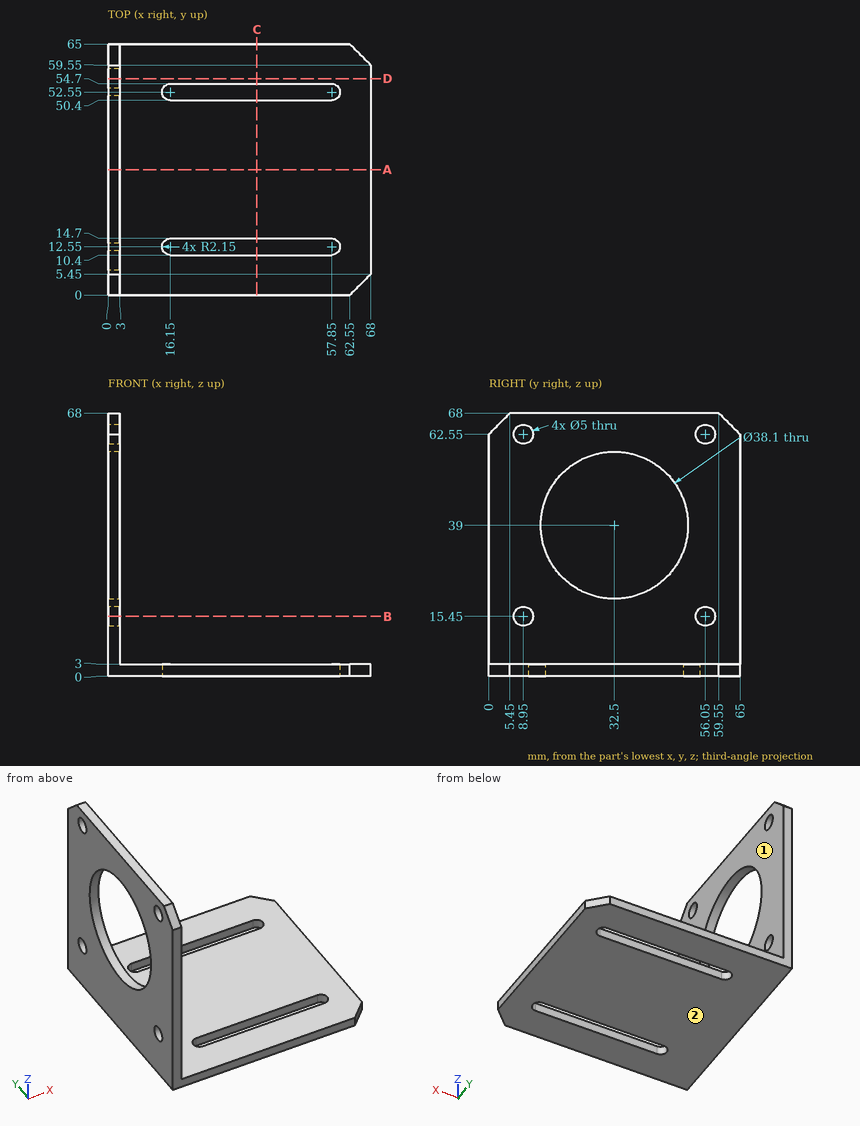
Study the drawing (mm; zero at the part's minimum x, y, z) and answer. A direction names the side the tool comes from. Give positions to 0.01 mm unless a question says otherwise; leave off trailing zeros. Loops run counter-clockwise (first coordinate to the right, second up) from the corner with the lowest first, then second, coordinate; pieces in that order, holes last. Notation, with made-up numbers: (47.25, 86) -> (106.25, 86) arc R13 ccw to (106.25, 91) -> close; hole circle Ø2 at (-9, -18). An arc over 180 degrees is marked (long way). Write item = value, one per line. Start each with the question number.
(1) Find the intervals of material crossed by probe 1 along Z at (x, y) = (1, 56.05); probe 2 along Y at (x, z) = (1.7, 62.55); probe 3 along Z at (x, y) = (2, 32.5), in increasing order. Write a range as from..to.
(2) Which of the six approach directions +Z, -Z, +X, -X, +Y, -Y give full straight-line access (tool end or side, diameter ignored) to the marked faces 1 and 2?
(3) Find section B-B on z = 15.45. Give the vertices of the cut face in (x, y).
(4) Given pin 1 Ø6 at (y, z) = (24, 17.5) entering from +X; pin 2 Ø4 at (y, z) = (8.95, 62.55) entering from -X, each flat-ended and moving along its own axis, determine where each tip first touches the part or whether it passes through.
(5) Find section A-A on y = 32.5. Give the vertices of the cut face in (x, z).
(6) Find section C-C on x = 38.5. Give the vertices of the cut face in (y, z).
(7) Find section D-D on y = 56.05. Give the vertices of the cut face in (x, z), and give its area (3 significant figures).
From the geometry:
q1.probe_1 = 0..12.95, 17.95..60.05, 65.05..68
q1.probe_2 = 0..6.45, 11.45..53.55, 58.55..65
q1.probe_3 = 0..19.95, 58.05..68
q2.face_1 = +Z, +X, +Y, -Y
q2.face_2 = -Z, +X, -X, +Y, -Y
q3.outline = (0, 0) -> (3, 0) -> (3, 6.45) -> (0, 6.45) -> close; (0, 11.45) -> (3, 11.45) -> (3, 53.55) -> (0, 53.55) -> close; (0, 58.55) -> (3, 58.55) -> (3, 65) -> (0, 65) -> close
q4.pin_1 = 3
q4.pin_2 = through
q5.outline = (0, 0) -> (68, 0) -> (68, 3) -> (3, 3) -> (3, 19.95) -> (0, 19.95) -> close; (0, 58.05) -> (3, 58.05) -> (3, 68) -> (0, 68) -> close
q6.outline = (0, 0) -> (10.4, 0) -> (10.4, 3) -> (0, 3) -> close; (14.7, 0) -> (50.4, 0) -> (50.4, 3) -> (14.7, 3) -> close; (54.7, 0) -> (65, 0) -> (65, 3) -> (54.7, 3) -> close
q7.outline = (0, 0) -> (68, 0) -> (68, 3) -> (3, 3) -> (3, 12.95) -> (0, 12.95) -> close; (0, 17.95) -> (3, 17.95) -> (3, 60.05) -> (0, 60.05) -> close; (0, 65.05) -> (3, 65.05) -> (3, 68) -> (0, 68) -> close
q7.area = 369 mm^2
